Study the drawing (mm; zero at the part's minimum x, y, z) and answer. A direction names the side the tool comes from. Round coordinates to 2 decimals unless told otherwise and drop trailing zeros. Loops run counter-clockwise (first coordinate to the right, second up) from the corner with the lowest first, then second, coordinate; pieces in that order, holes last. Notation, with made-up numbers: (-20.5, 19) - (-14.5, 19) arc R37 ccw to (-14.5, 56) - close; hole circle Ø8 at (76, 61). An arc over 180 degrees is marked (long way). One line per item, written item: value.
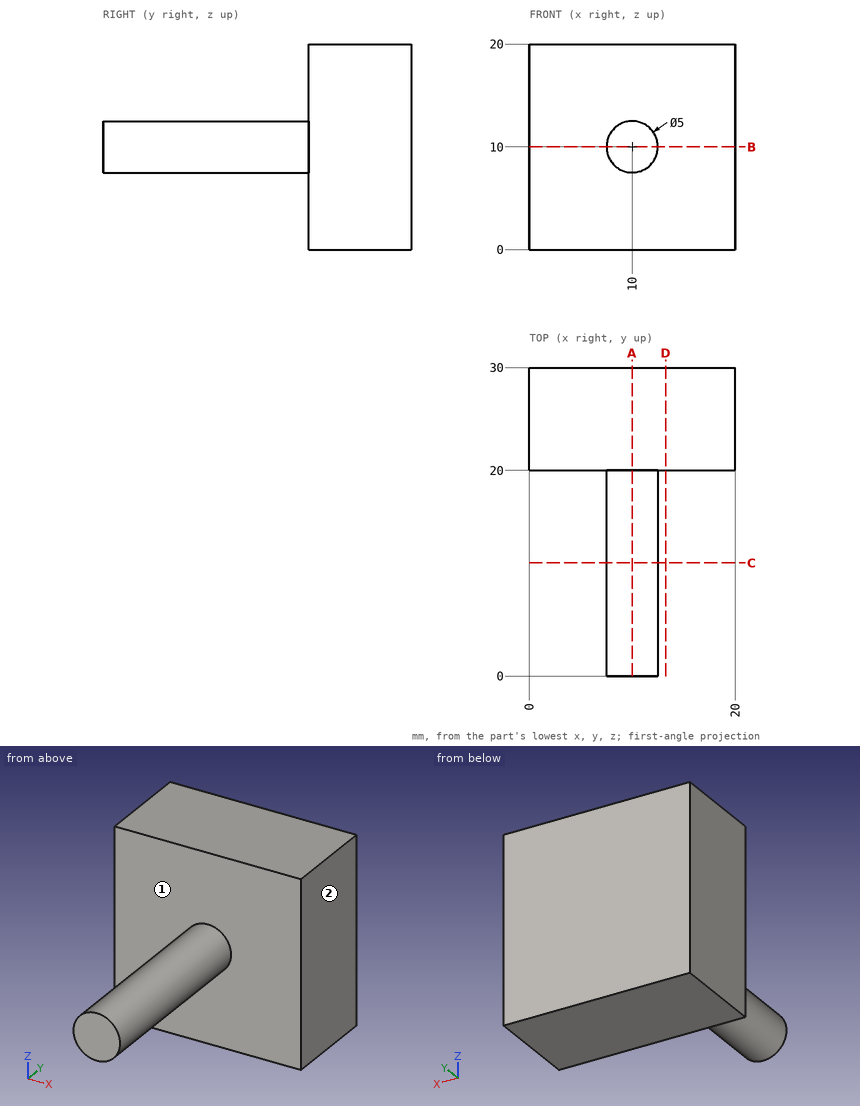
1) A cutting plane is placed at D-D on x = 13.25. Give the vertices of the cut face in (y, z), and give its area (3 significant figures).
Final values:
outline: (20, 0) - (30, 0) - (30, 20) - (20, 20) - close
area: 200 mm2
2) For the marked faces 1 and 2, determine the directions among +Z, -Z, +X, -X, +Y, -Y from which every point of the face is accessible in a straight line to the end or side of a thin tool.
Final values:
face 1: -Y
face 2: +Z, -Z, +X, +Y, -Y
3) A cutting plane is placed at B-B on z = 10. Give the vertices of the cut face in (x, y), and give its area (3 significant figures).
Final values:
outline: (0, 20) - (7.5, 20) - (7.5, 0) - (12.5, 0) - (12.5, 20) - (20, 20) - (20, 30) - (0, 30) - close
area: 300 mm2
4) A cutting plane is placed at C-C on y = 11. Give the vertices of the cut face in (x, z).
Final values:
outline: circle Ø5 at (10, 10)
5) A cutting plane is placed at A-A on x = 10. Give the vertices of the cut face in (y, z), and give its area (3 significant figures).
Final values:
outline: (0, 7.5) - (20, 7.5) - (20, 0) - (30, 0) - (30, 20) - (20, 20) - (20, 12.5) - (0, 12.5) - close
area: 300 mm2
6) Consider L1, parallel to Y at x = 16.25, z = 1; L2, parallel to Z at x = 9.5, y = 5.5; L3, parallel to X at y = 9.25, z = 10.25. Determine where each line is inside the solid, lowest interval first.
Final values:
L1: 20 to 30
L2: 7.55 to 12.45
L3: 7.51 to 12.49
7) Each of these flat-tipped pins is pushed along its axis until it touches: pin 1 Ø3 at (x, z) = (15.5, 17.5) entering from -Y; pin 2 Ø8 at (x, y) = (13, 12.5) entering from -Z; pin 3 Ø3 at (x, y) = (5.5, 15.5) entering from -Z; pin 4 Ø2 at (y, z) = (5, 10.5) entering from -X. Where does it stop, or does it pass through?
Final values:
pin 1: y = 20
pin 2: z = 7.5
pin 3: through
pin 4: x = 7.5
